```python
from build123d import *

# Parameters (mm, degrees)
SKETCH_1_W                  = 160
SKETCH_1_H                  = 160
EXTRUDE_1_DEPTH             = 2.5
SKETCH_2_R                  = 5
CUT_EXTRUDE_1_DEPTH         = 227.287980238
PATTERN_LINEAR_1_COUNT      = 2
PATTERN_LINEAR_1_PITCH      = 80
PATTERN_LINEAR_1_COUNT_DIR2 = 2
PATTERN_LINEAR_1_PITCH_DIR2 = 80


with BuildPart() as part:
    # 草图1 → 凸台-拉伸1 (new body)
    with BuildSketch(Plane.XY):
        with Locations((80, 80)):
            Rectangle(SKETCH_1_W, SKETCH_1_H)
    extrude(amount=EXTRUDE_1_DEPTH)

    # 草图2 → 切除-拉伸1 (cut, through all)
    with BuildSketch(Plane.XY.offset(2.5)):
        with Locations((40, 120)):
            Circle(SKETCH_2_R)
    cut_extrude_1 = extrude(amount=-CUT_EXTRUDE_1_DEPTH, mode=Mode.SUBTRACT)

    # 阵列(线性)1: Cut-Extrude 1 2 × 2
    with Locations(*[(i * PATTERN_LINEAR_1_PITCH, -j * PATTERN_LINEAR_1_PITCH_DIR2, 0) for i in range(PATTERN_LINEAR_1_COUNT) for j in range(PATTERN_LINEAR_1_COUNT_DIR2) if (i, j) != (0, 0)]):
        add(cut_extrude_1, mode=Mode.SUBTRACT)


solid = part.part
```
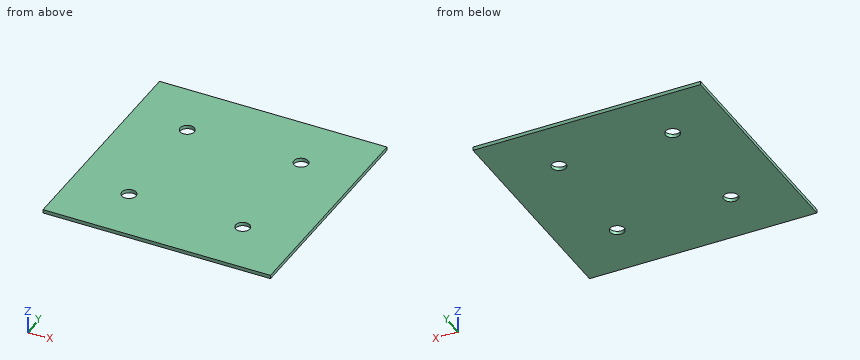
Source: CAD feature listing. Evaluate the final solid. Frame: model axes, mm. Give positions to 0.01 mm unless a question says otherwise; leave off trailing zeros. Order: outer loops, then holes, each group sorted by start corner. A loop starts at its lowest first (then second) coordinate and runs counter-clockwise, first axis right, second up.
(1) Material intervals for line 1 along Y through (x, z) = (120, 0.7); line 2 along Y through (x, z) = (39, 1.3); line 3 along X through (y, z) = (43, 0.8), sorted ascending.
(2) Section query A-A (x = 40). Return the cut outline in (y, z), plus the area to 3 significant figures.
(3) Contact query for a flat-ended pin moving along its axis: P1, Ø13, axis at x = 120, y = 120, coming from the +Z side. Output: stop coordinate, or through.
Outcome:
1. line 1: y = 0 to 35, 45 to 115, 125 to 160
1. line 2: y = 0 to 35.1, 44.9 to 115.1, 124.9 to 160
1. line 3: x = 0 to 36, 44 to 116, 124 to 160
2. outline: (0, 0) - (35, 0) - (35, 2.5) - (0, 2.5) - close; (45, 0) - (115, 0) - (115, 2.5) - (45, 2.5) - close; (125, 0) - (160, 0) - (160, 2.5) - (125, 2.5) - close
2. area: 350 mm2
3. P1: stops at z = 2.5
